from build123d import *

# Parameters (mm, degrees)
SKETCH_1_W          = 1658
SKETCH_1_H          = 338
EXTRUDE_1_DEPTH     = 1.5
SKETCH_2_W          = 1658
SKETCH_2_H          = 338
SKETCH_2_W_2        = 1655
SKETCH_2_H_2        = 335
EXTRUDE_2_DEPTH     = 15
SKETCH_3_W          = 1658
SKETCH_3_H          = 338
SKETCH_3_W_2        = 1638
SKETCH_3_H_2        = 318
EXTRUDE_3_DEPTH     = 1.5
SKETCH_5_R          = 2.5
SKETCH_5_R_2        = 1
EXTRUDE_4_DEPTH     = 6
SKETCH_6_R          = 3
CUT_EXTRUDE_1_DEPTH = 19
FILLET_1_R          = 1


with BuildPart() as part:
    # 草图1 → 凸台-拉伸1 (new body)
    with BuildSketch(Plane.XY):
        Rectangle(SKETCH_1_W, SKETCH_1_H)
    extrude(amount=EXTRUDE_1_DEPTH)

    # 草图2 → 凸台-拉伸2 (add)
    with BuildSketch(Plane(origin=(0, 0, 0), x_dir=(-1, 0, 0), z_dir=(0, 0, -1))):
        Rectangle(SKETCH_2_W, SKETCH_2_H)
        Rectangle(SKETCH_2_W_2, SKETCH_2_H_2, mode=Mode.SUBTRACT)
    extrude(amount=EXTRUDE_2_DEPTH)

    # 草图3 → 凸台-拉伸3 (add)
    with BuildSketch(Plane(origin=(0, 0, -15), x_dir=(-1, 0, 0), z_dir=(0, 0, -1))):
        Rectangle(SKETCH_3_W, SKETCH_3_H)
        Rectangle(SKETCH_3_W_2, SKETCH_3_H_2, mode=Mode.SUBTRACT)
    extrude(amount=EXTRUDE_3_DEPTH)

    # 草图5 → 凸台-拉伸4 (add)
    with BuildSketch(Plane(origin=(0, 169, 0), x_dir=(1, 0, 0), z_dir=(0, 1, 0))):
        with Locations((240, 7.5)):
            Circle(SKETCH_5_R)
        with Locations((240, 7.5)):
            Circle(SKETCH_5_R_2, mode=Mode.SUBTRACT)
        with Locations((-240, 7.5)):
            Circle(SKETCH_5_R)
        with Locations((-240, 7.5)):
            Circle(SKETCH_5_R_2, mode=Mode.SUBTRACT)
    extrude(amount=EXTRUDE_4_DEPTH)

    # 草图6 → 切除-拉伸1 (cut, through all)
    with BuildSketch(Plane.XY.offset(1.5)):
        with Locations((-800, -140)):
            Circle(SKETCH_6_R)
        with Locations((800, -140)):
            Circle(SKETCH_6_R)
    extrude(amount=-CUT_EXTRUDE_1_DEPTH, mode=Mode.SUBTRACT)

    # 圆角1
    fillet_1_edges = [part.edges().sort_by_distance(p)[0] for p in [
        (829, 0, 1.5),
        (0, 169, 1.5),
        (-829, 0, -16.5),
        (0, 169, -16.5),
        (829, 0, -16.5),
        (0, -169, -16.5),
        (-829, 0, 1.5),
        (0, -169, 1.5),
        (-829, 169, -7.5),
        (829, 169, -7.5),
        (829, -169, -7.5),
        (-829, -169, -7.5),
    ]]
    fillet(fillet_1_edges, radius=FILLET_1_R)


solid = part.part
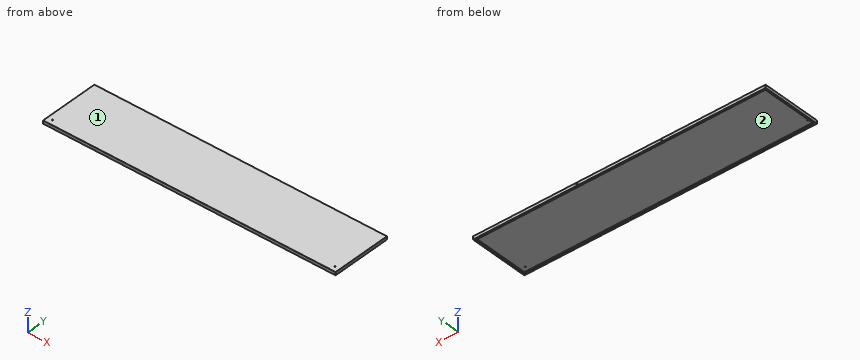
Verification items for the finished model (mm, model axes). Face numbers are marked on the shaded views. Give positions to 0.01 mm unless a question says otherwise; leave off trailing zeros. Loops run counter-clockwise (first coordinate to the right, second up) from the corner with the lowest first, then second, coordinate; pieces in that order, holes last. Notation, with made-up numbers: (73.5, 63.25) - (102.5, 63.25) arc R22 ccw to (102.5, 84.25) - close; hole circle Ø1 at (16, 74). An arc over 180 degrees is marked (long way). Write item = value, one per line. Start each with the question number.
Q1. Thickness scan on line 1 (X direction, y = 171.1, z = -7.5); line 2 (X direction, y = -140, z = 1.2); line 3 (Y direction, x = 452.5, z = -2.25). Record the ranges inside material, lowest first.
Q2. Cross-section at B-B, the plane x = -708.5. Enter the section's corners in (y, z), and give its area (3 significant figures).
Q3. Depth check by flat-ended pin: P1, Ø1, axis at x = 240, z = -7.5, coming from the +Y side; P2, Ø12, axis at x = 360.5, y = -20.5, coming from the -Z side. Enter the tip coordinate at first touch or a pass-through.
Q4. Mould release check, pull along X, two halves, no side actions. Record for the marked faces 1 and 2: released by +X, released by -X, zero draft, split by the parting line, or undercut.
Q5. Cross-section at A-A, the plane y = -56.5. Enter the section's corners in (x, z).
Answer key:
q1.line_1 = -242.5 to -241, -239 to -237.5, 237.5 to 239, 241 to 242.5
q1.line_2 = -828.71 to -803, -797 to 797, 803 to 828.71
q1.line_3 = -169 to -167.5, 167.5 to 169
q2.outline = (-169, -15.5) arc R1 ccw to (-168, -16.5) - (-159, -16.5) - (-159, -15) - (-167.5, -15) - (-167.5, 0) - (167.5, 0) - (167.5, -15) - (159, -15) - (159, -16.5) - (168, -16.5) arc R1 ccw to (169, -15.5) - (169, 0.5) arc R1 ccw to (168, 1.5) - (-168, 1.5) arc R1 ccw to (-169, 0.5) - close
q2.area = 581 mm^2
q3.P1 = 169
q3.P2 = 0
q4.face_1 = zero draft
q4.face_2 = undercut
q5.outline = (-829, -15.5) arc R1 ccw to (-828, -16.5) - (-819, -16.5) - (-819, -15) - (-827.5, -15) - (-827.5, 0) - (827.5, 0) - (827.5, -15) - (819, -15) - (819, -16.5) - (828, -16.5) arc R1 ccw to (829, -15.5) - (829, 0.5) arc R1 ccw to (828, 1.5) - (-828, 1.5) arc R1 ccw to (-829, 0.5) - close
